```python
from build123d import *

# Parameters (mm, degrees)
SKETCH011_W     = 84
SKETCH011_H     = 54
SKETCH011_R     = 6
SKETCH011_W_2   = 3
SKETCH011_H_2   = 25
PAD004_DEPTH    = 2
SKETCH012_W     = 84
SKETCH012_H     = 54
SKETCH012_W_2   = 80
SKETCH012_H_2   = 50
PAD005_DEPTH    = 38
SKETCH013_W     = 76
SKETCH013_H     = 2.2
POCKET007_DEPTH = 54.001


with BuildPart() as part:
    # Sketch011 (on XY_Plane005 of Origin010) → Pad004 (new body)
    with BuildSketch(Plane.XY):
        with Locations((42, -27)):
            Rectangle(SKETCH011_W, SKETCH011_H)
        with Locations((25.609009, -11.632301)):
            Circle(SKETCH011_R, mode=Mode.SUBTRACT)
        with Locations((25.479133, -35.686392)):
            Rectangle(SKETCH011_W_2, SKETCH011_H_2, mode=Mode.SUBTRACT)
    extrude(amount=PAD004_DEPTH)

    # Sketch012 (on Face11 of Pad004) → Pad005 (join)
    with BuildSketch(Plane.XY.offset(2)):
        with Locations((42, -27)):
            Rectangle(SKETCH012_W, SKETCH012_H)
        with Locations((42, -27)):
            Rectangle(SKETCH012_W_2, SKETCH012_H_2, mode=Mode.SUBTRACT)
    extrude(amount=PAD005_DEPTH)

    # Sketch013 (on Face14 of Pad005) → Pocket007 (cut, through all)
    with BuildSketch(Plane(origin=(0, 0, 0), x_dir=(-1, 0, 0), z_dir=(0, 1, 0))):
        with Locations((-43, 35.1)):
            Rectangle(SKETCH013_W, SKETCH013_H)
    extrude(amount=-POCKET007_DEPTH, mode=Mode.SUBTRACT)


solid = part.part
```
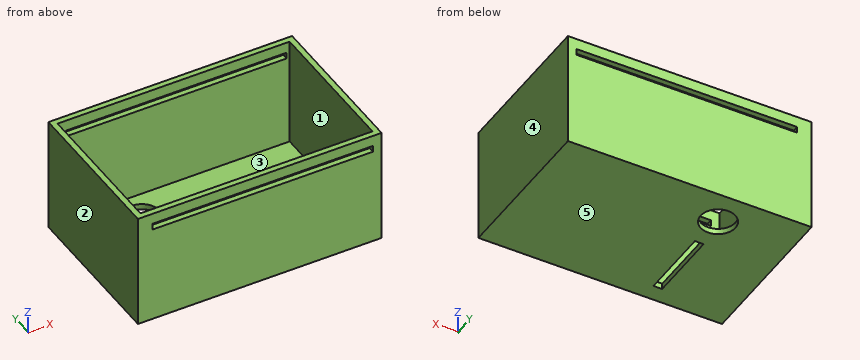
Source: CAD feature listing. Evaluate the final solid. Frame: model axes, mm. Face numbers are marked on the shaded views. A direction names the side the tool comes from. Round coordinates to 2 decimals unless told otherwise and drop trailing zeros. Write each loop counter-clockwise with the first axis right and the second up, starting at its lowest first coordinate (ties: lowest second). Pieces come first, ordered by that corner, then holes. Notation, with made-up numbers: M 64.5,33 L 93.5,33 A20 cw 93.5,59 Z; hole C 5.25,-25.75 d7. An arc over 180 degrees is marked long. Use CSV: the item, a comma, the result in double quotes. Start each with the question number.
Q1. Pull-direction query (X, two-part tool) for the marked faces 3, 4 and 5; classes: +X half, -X half, draft (parallel to the pull), parting line (faces both ways), or undercut.
Q2. Cut plane B-B on y = -38. Output: boundary loops of the cut face in (x, z).
Q3. Cut plane A-A on z = 23. Output: boundary loops of the cut face in (x, y).
Q4. Line query: line 1 (X direction, y = -34, z = 5); line 2 (Y direction, x = 12, z = 18); line 3 (Z direction, x = 21.5, y = -36). Output: solid intervals per line, ascending. Write a range as from..to.
Q5. First-contact query: P1, Ø9.5, axis at x = 25.61, y = -11.63, coming from the -Z side; P2, Ø15, axis at x = 35.5, y = -18.5, coming from the +Z side. Flat tips, straight axial feed; report the tip coordinate or a pass-through.
Q6. Cut plane C-C on x = 14. Output: boundary loops of the cut face in (y, z), plus the area to 3 significant figures.
Q7. Cut plane D-D on y = -3.5. Output: boundary loops of the cut face in (x, z), plus the area to 3 significant figures.
Q8. Access query for the marked faces 1 and 2. Directions: +Z, -Z, +X, -X, +Y, -Y. A direction counts if a zero-diameter tool reaches every point of the face in a straight line with its end or side. Return the directions, or none.
Results found:
1,face 3,"undercut"
1,face 4,"+X half"
1,face 5,"draft"
2,outline,"M 0,0 L 23.98,0 L 23.98,2 L 2,2 L 2,40 L 0,40 Z; M 26.98,0 L 84,0 L 84,40 L 82,40 L 82,2 L 26.98,2 Z"
3,outline,"M 0,-54 L 84,-54 L 84,0 L 0,0 Z; hole M 2,-52 L 82,-52 L 82,-2 L 2,-2 Z"
4,line 1,"0..2, 82..84"
4,line 2,"-54..-52, -2..0"
4,line 3,"0..2"
5,P1,"through"
5,P2,"z = 2"
6,outline,"M -54,0 L 0,0 L 0,34 L -2,34 L -2,2 L -52,2 L -52,34 L -54,34 Z; M -54,36.2 L -52,36.2 L -52,40 L -54,40 Z; M -2,36.2 L 0,36.2 L 0,40 L -2,40 Z"
6,area,"251 mm^2"
7,outline,"M 0,0 L 84,0 L 84,40 L 82,40 L 82,2 L 2,2 L 2,40 L 0,40 Z"
7,area,"320 mm^2"
8,face 1,"+Z"
8,face 2,"+Z, -Z, -X, +Y, -Y"
